Check sheet for the modelled part. Datum: model origin and axes. Units: mm. Face numbers are marked on the shaded views. A direction names the side the tool comes from. Give positions to 0.01 mm unless a question says otherwise; leave off trailing zeros. Order: outer loops, then holes, each group sorted by start corner. A loop starts at its lowest first (then second) coordinate and runs counter-clockwise, first axis right, second up.
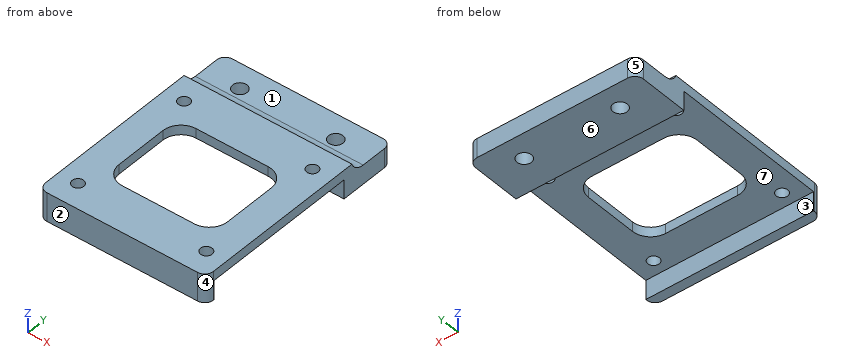
from build123d import *

# Parameters (mm, degrees)
SKETCH1_W           = 44.45
SKETCH1_H           = 59.4
SKETCH1_R           = 1.905
SKETCH1_R_2         = 1.524
BOSS_EXTRUDE1_DEPTH = 5.08
SKETCH2_W           = 44.45
SKETCH2_H           = 46.7
SKETCH2_R           = 1.524
BOSS_EXTRUDE2_DEPTH = 2.54
SKETCH3_W           = 44.45
SKETCH3_H           = 41.62
CUT_EXTRUDE1_DEPTH  = 5.08
FILLET2_R           = 2.286
SKETCH4_W           = 28.72406321
SKETCH4_H           = 23.663865546
CUT_EXTRUDE2_DEPTH  = 64.969700054
FILLET3_R           = 4.826
FILLET4_R           = 3.81


with BuildPart() as part:
    # Sketch1 → Boss-Extrude1 (new body)
    with BuildSketch(Plane.XY):
        with Locations((12.7, -23.35)):
            Rectangle(SKETCH1_W, SKETCH1_H)
        Circle(SKETCH1_R, mode=Mode.SUBTRACT)
        with Locations((25.4, 0)):
            Circle(SKETCH1_R, mode=Mode.SUBTRACT)
        with Locations((-4.3, -12.7)):
            Circle(SKETCH1_R_2, mode=Mode.SUBTRACT)
        with Locations((29.7, -12.7)):
            Circle(SKETCH1_R_2, mode=Mode.SUBTRACT)
        with Locations((29.7, -46.7)):
            Circle(SKETCH1_R_2, mode=Mode.SUBTRACT)
        with Locations((-4.3, -46.7)):
            Circle(SKETCH1_R_2, mode=Mode.SUBTRACT)
    extrude(amount=BOSS_EXTRUDE1_DEPTH)

    # Sketch2 → Boss-Extrude2 (add)
    with BuildSketch(Plane.XY.offset(5.08)):
        with Locations((12.7, -29.7)):
            Rectangle(SKETCH2_W, SKETCH2_H)
        with Locations((-4.3, -12.7)):
            Circle(SKETCH2_R, mode=Mode.SUBTRACT)
        with Locations((-4.3, -46.7)):
            Circle(SKETCH2_R, mode=Mode.SUBTRACT)
        with Locations((29.7, -12.7)):
            Circle(SKETCH2_R, mode=Mode.SUBTRACT)
        with Locations((29.7, -46.7)):
            Circle(SKETCH2_R, mode=Mode.SUBTRACT)
    extrude(amount=BOSS_EXTRUDE2_DEPTH)

    # Sketch3 → Cut-Extrude1 (cut)
    with BuildSketch(Plane(origin=(0, 0, 0), x_dir=(-1, 0, 0), z_dir=(0, 0, -1))):
        with Locations((-12.7, -29.7)):
            Rectangle(SKETCH3_W, SKETCH3_H)
    extrude(amount=-CUT_EXTRUDE1_DEPTH, mode=Mode.SUBTRACT)

    # Fillet2
    fillet2_edges = [part.edges().sort_by_distance(p)[0] for p in [
        (-9.525, 6.35, 2.54),
        (34.925, 6.35, 2.54),
        (34.925, -53.05, 3.81),
        (-9.525, -53.05, 3.81),
    ]]
    fillet(fillet2_edges, radius=FILLET2_R)

    # Sketch4 → Cut-Extrude2 (cut, through all)
    with BuildSketch(Plane.XY.offset(7.62)):
        with Locations((12.7, -29.7)):
            Rectangle(SKETCH4_W, SKETCH4_H)
    extrude(amount=-CUT_EXTRUDE2_DEPTH, mode=Mode.SUBTRACT)

    # Fillet3
    fillet3_edges = [part.edges().sort_by_distance(p)[0] for p in [
        (-1.662031605, -41.531932773, 6.35),
        (-1.662031605, -17.868067227, 6.35),
        (27.062031605, -17.868067227, 6.35),
        (27.062031605, -41.531932773, 6.35),
    ]]
    fillet(fillet3_edges, radius=FILLET3_R)

    # Fillet4
    # the kernel refuses this fillet: 3.81 mm, written as the material it adds along each edge
    with BuildSketch(Plane(origin=(34.925, -6.35, 5.08), x_dir=(0, 0, 1), z_dir=(-1, 0, 0))) as fillet4_piece_1:
        with BuildLine():
            CenterArc((3.81, 3.592102448), FILLET4_R, 180, 70.528779366)
            Line((0, 3.592102448), (-0.0762, 3.592102448))
            Line((-0.0762, 3.592102448), (-0.0762, 0))
            Line((-0.0762, 0), (0, -0.0762))
            ThreePointArc((0, -0.0762), (1.27, -0.0762), (2.5146, -0.071842049))
            Line((2.5146, -0.071842049), (2.54, 0))
        make_face()
    extrude(amount=44.45)


solid = part.part
1) Section check D-D, the plane y = -28.5. Record the cut outline in (x, z) (3 decimals).
Recorded:
outline: (-9.525, 5.08) - (-1.662, 5.08) - (-1.662, 7.62) - (-9.525, 7.62) - close; (27.062, 5.08) - (34.925, 5.08) - (34.925, 7.62) - (27.062, 7.62) - close
2) Depth check by flat-ended pin: pin 1 Ø2.5 at (x, y) = (-4.3, -46.7) entering from -Z; pin 2 Ø1.5 at (x, z) = (11.5, 6.5) entering from +Y; pin 3 Ø5 at (x, y) = (29.7, -46.7) entering from -Z; pin 4 Ø2.5 at (x, y) = (18.5, 0) entering from +Z. Enter the tip coordinate at first touch or a pass-through.
Recorded:
pin 1: passes through
pin 2: stops at y = -4.92
pin 3: stops at z = 5.08
pin 4: stops at z = 5.08
3) Section check A-A, the plane y = -46.7. Record the cut outline in (x, z) (3 decimals), then the cut area to 3 significant figures.
Recorded:
outline: (-9.525, 5.08) - (-5.824, 5.08) - (-5.824, 7.62) - (-9.525, 7.62) - close; (-2.776, 5.08) - (28.176, 5.08) - (28.176, 7.62) - (-2.776, 7.62) - close; (31.224, 5.08) - (34.925, 5.08) - (34.925, 7.62) - (31.224, 7.62) - close
area: 97.4 mm2
4) Section check B-B, the plane z = 1.25. Record the cut outline in (x, y) (3 decimals).
Recorded:
outline: (-9.525, -50.764) arc R2.286 ccw to (-7.239, -53.05) - (32.639, -53.05) arc R2.286 ccw to (34.925, -50.764) - (34.925, -50.51) - (-9.525, -50.51) - close; (-9.525, -8.89) - (34.925, -8.89) - (34.925, 4.064) arc R2.286 ccw to (32.639, 6.35) - (-7.239, 6.35) arc R2.286 ccw to (-9.525, 4.064) - close; hole circle Ø3.81 at (0, 0); hole circle Ø3.81 at (25.4, 0)
5) Draft check along Y on the marked faces 4, 5, 6 and 7. Enter one of: +Y half, -Y half, draft (parallel to the pull), parting line (faces both ways), or undercut.
Recorded:
face 4: -Y half
face 5: +Y half
face 6: draft
face 7: undercut
6) Section check C-C, the plane x = 29.7. Record the cut outline in (y, z).
Recorded:
outline: (-53.05, 0) - (-50.51, 0) - (-50.51, 5.08) - (-48.22, 5.08) - (-48.22, 7.62) - (-53.05, 7.62) - close; (-45.18, 5.08) - (-14.22, 5.08) - (-14.22, 7.62) - (-45.18, 7.62) - close; (-11.18, 5.08) - (-8.89, 5.08) - (-8.89, 0) - (6.35, 0) - (6.35, 5.08) - (-2.76, 5.08) arc R3.81 cw to (-6.35, 7.62) - (-11.18, 7.62) - close
7) Material ranges on L1, parallel to Y at x = 25.4, z = 3 (3 decimals); L2, parallel to X at y = -12.7, z = 6.2 (3 decimals); L3, parallel to Y at x = 20.5, z = 1.5, recorded low to high.
Recorded:
L1: y = -53.05 to -50.51, -8.89 to -1.905, 1.905 to 6.35
L2: x = -9.525 to -5.824, -2.776 to 28.176, 31.224 to 34.925
L3: y = -53.05 to -50.51, -8.89 to 6.35
8) Set-up check for the marked faces 1, 2 and 3: record each of +Z, -Z, +X, -X, +Y, -Y from which the full face is reachable in a straight line by a thin tool's end or side.
Recorded:
face 1: +Z, +X, -X, +Y
face 2: +Z, -Z, +X, -X, -Y
face 3: -Z, +X, -X
